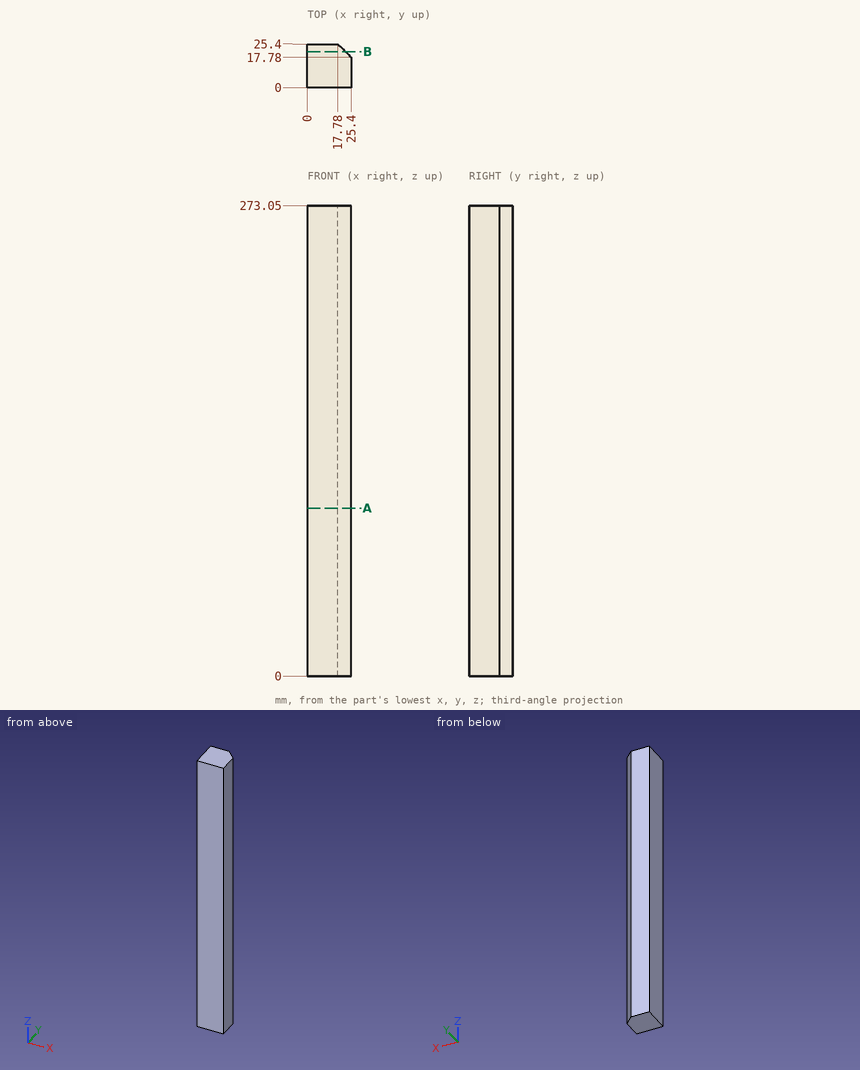
Job drawing, mm, ordinate dimensions from the low corner. One solid piece. Round coordinates to 2 decimals unless told otherwise and drop trailing zeros. Loops run counter-clockwise (first coordinate to the right, second up) from the corner with the lowest first, then second, coordinate; pieces in that order, holes last. Notation, with made-up numbers: M 52.5,76.25 L 59.5,76.25 A18 cw 59.5,109.25 Z; hole C 20,35.5 d8. An arc over 180 degrees is marked long. One line per question, with ' | ' between items. Start each with the question number.
Item 1: Cut at B-B, the plane y = 21. Write the cut outline in (x, z).
Item 2: Cut at A-A, the plane z = 97.5. Write the cut outline in (x, y), plus the area to 3 significant figures.
Item 3: Pin check, flat tip, straight feed: pin 1 Ø1 at (y, z) = (12.5, 65.5) entering from -X. Stop position of the tip, or through.
Item 4: Wall check: line 1 (Y direction, x = 18.25, z = 80); line 2 (X direction, y = 19.75, z = 151). Give the ranges that are in metal, low to high.
Responses:
1) outline: M 0,0 L 22.18,0 L 22.18,273.05 L 0,273.05 Z
2) outline: M 0,0 L 25.4,0 L 25.4,17.78 L 17.78,25.4 L 0,25.4 Z | area: 616 mm²
3) pin 1: stops at x = 0
4) line 1: y = 0 to 24.93 | line 2: x = 0 to 23.43
